```python
from build123d import *

# Parameters (mm, degrees)
SKETCH1_R           = 31
SKETCH1_R_2         = 25
BOSS_EXTRUDE1_DEPTH = 1157
SKETCH2_W           = 180
SKETCH2_H           = 75
SKETCH2_R           = 8
BOSS_EXTRUDE2_DEPTH = 12
SKETCH3_W           = 200
SKETCH3_H           = 150
BOSS_EXTRUDE3_DEPTH = 16


with BuildPart() as part:
    # Sketch1 → Boss-Extrude1 (new body)
    with BuildSketch(Plane.XY):
        Circle(SKETCH1_R)
        Circle(SKETCH1_R_2, mode=Mode.SUBTRACT)
    extrude(amount=BOSS_EXTRUDE1_DEPTH)

    # Sketch2 → Boss-Extrude2 (add)
    with BuildSketch(Plane(origin=(0, 0, 0), x_dir=(-1, 0, 0), z_dir=(0, 0, -1))):
        Rectangle(SKETCH2_W, SKETCH2_H)
        with Locations((64.227589169, 0)):
            Circle(SKETCH2_R, mode=Mode.SUBTRACT)
        with Locations((-68.030538528, 0)):
            Circle(SKETCH2_R, mode=Mode.SUBTRACT)
    extrude(amount=BOSS_EXTRUDE2_DEPTH)

    # Sketch3 → Boss-Extrude3 (add)
    with BuildSketch(Plane.XY.offset(1157)):
        Rectangle(SKETCH3_W, SKETCH3_H)
        with BuildLine():
            Line((-42, 25), (-42, -25))
            ThreePointArc((-42, -25), (-50, -33), (-58, -25))
            Line((-58, -25), (-58, 25))
            ThreePointArc((-58, 25), (-50, 33), (-42, 25))
        make_face(mode=Mode.SUBTRACT)
        with BuildLine():
            Line((42, 25), (42, -25))
            ThreePointArc((42, -25), (50, -33), (58, -25))
            Line((58, -25), (58, 25))
            ThreePointArc((58, 25), (50, 33), (42, 25))
        make_face(mode=Mode.SUBTRACT)
    extrude(amount=BOSS_EXTRUDE3_DEPTH)


solid = part.part
```
Model file for the job. Use its own axes, mm. A direction names the side the tool comes from. Coordinates: 2 decimals unless noted, no trailing zeros. Write each loop counter-clockwise with the first axis right and the second up, starting at its lowest first coordinate (ties: lowest second). Pieces come first, ordered by that corner, then holes. Notation, with made-up numbers: (-33, 76.25) - (3, 76.25) arc R22 ccw to (3, 83.25) - close; hole circle Ø10 at (20, -28). An arc over 180 degrees is marked (long way). Use a Markdown table: item, result. Add a question column.
Item 1: Band-saw the part on B-B, the plane y = -61. Write the cut outline in (x, z).
Item 2: Drill centre lines: line 1 along Y through (x, z) = (0, 481); line 2 along X through (y, z) = (3, 701); line 3 along Z through (x, y) = (71, 19). Where is each one in solid material? Low to high.
Item 3: Band-saw the part on A-A, the plane z = 402.5. Write the cut outline in (x, y).
Item 4: Two-plate mould, pull along Y, no slides. Class faces 3 (the face through (21, 26, 0)), 4 (the face through (0, 0, 1157)), 5 (the face through (-4.036, 30.736, 570.401)), 6 (the face through (23.846, 7.509, 570.401)): pulls with the +Y half, pulls with the -Y half, needs draft (parallel to the pull), parting line crosses it, or undercut.
Item 5: Drop flat-ended pins along their axis: pin 1 (1 mm diameter, centred on x = -12, z = 933, fed in from +Y); pin 2 (13 mm diameter, centred on y = 4, z = -7, fed in from -X); pin 3 (8 mm diameter, centred on y = 18, z = 693.5, fed in from -X). Give the stop position or say it passes through.
Item 6: 3-axis set-ups, long thin cutter, end or side, ignore diameter. For faces 1 (the face through (1, 1, -12)), 2 (the face through (0, 0, 0)): which of +Z, -Z, +X, -X, +Y, -Y reach the whole face in a straight line?
A:
| question | item | result |
|---|---|---|
| 1 | outline | (-100, 1157) - (100, 1157) - (100, 1173) - (-100, 1173) - close |
| 2 | line 1 | y = -31 to -25, 25 to 31 |
| 2 | line 2 | x = -30.85 to -24.82, 24.82 to 30.85 |
| 2 | line 3 | z = -12 to 0, 1157 to 1173 |
| 3 | outline | circle Ø62 at (0, 0); hole circle Ø50 at (0, 0) |
| 4 | face 3 | needs draft |
| 4 | face 4 | undercut |
| 4 | face 5 | parting line crosses it |
| 4 | face 6 | undercut |
| 5 | pin 1 | stops at y = 28.79 |
| 5 | pin 2 | stops at x = -90 |
| 5 | pin 3 | stops at x = -27.66 |
| 6 | face 1 | -Z, +X, -X, +Y, -Y |
| 6 | face 2 | none |
